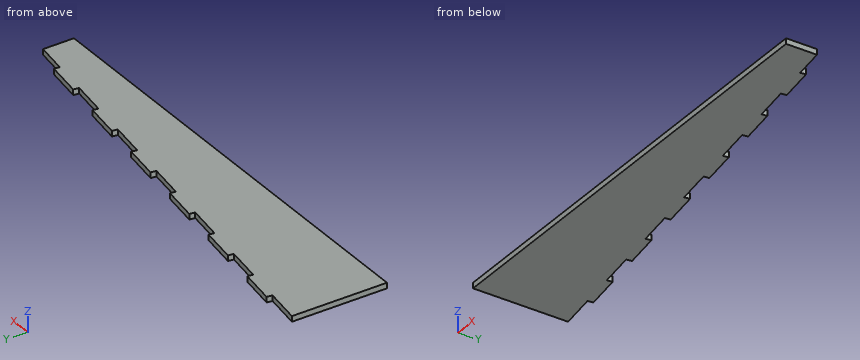
```python
from build123d import *

# Parameters (mm, degrees)
BOSS_EXTRU_1_DEPTH      = 3
ENL_V_MAT_EXTRU_1_DEPTH = 4


with BuildPart() as part:
    # Esquisse1 → Boss.-Extru.1 (new body)
    with BuildSketch(Plane.XY):
        Polygon((0, 0), (-255, 0), (-255, 55), (0, 19.9375), align=None)
    extrude(amount=BOSS_EXTRU_1_DEPTH)

    # Esquisse2 → Enlèv. mat.-Extru.1 (cut, through all)
    with BuildSketch(Plane.XY.offset(3)):
        Polygon((-235.186423203, 49.247406605), (-234.777768182, 52.219443125), (-255, 55), (-255, 51.971773415), align=None)
        Polygon((-195.150614588, 46.770709506), (-214.964191385, 49.495076315), (-215.372846406, 46.523039796), (-195.559269609, 43.798672986), align=None)
        Polygon((-155.523460994, 41.321975887), (-175.337037791, 44.046342696), (-175.745692812, 41.074306177), (-155.932116015, 38.349939367), align=None)
        Polygon((-115.8963074, 35.873242268), (-135.709884197, 38.597609077), (-136.118539219, 35.625572558), (-116.304962422, 32.901205748), align=None)
        Polygon((-76.269153806, 30.424508648), (-96.082730603, 33.148875458), (-96.491385625, 30.176838938), (-76.677808828, 27.452472129), align=None)
        Polygon((-36.642000213, 24.975775029), (-56.45557701, 27.700141839), (-56.864232031, 24.728105319), (-37.050655234, 22.00373851), align=None)
        Polygon((0, 19.9375), (-16.828423416, 22.25140822), (-17.237078437, 19.2793717), (0, 16.909273415), align=None)
    extrude(amount=-ENL_V_MAT_EXTRU_1_DEPTH, mode=Mode.SUBTRACT)


solid = part.part
```
Work out the finished part from the listing and answer in its coordinate system (mm). Coordinates: 2 decimals unless noted, no trailing zeros. Loops run counter-clockwise (first coordinate to the right, second up) from the corner with the lowest first, then second, coordinate; pieces in that order, holes last. Notation, with made-up numbers: M 84,47 L 104,47 A11 ccw 104,63 Z; hole C 54.5,40 d8. An arc over 180 degrees is marked long. Use CSV: the item, a comma, the result in double quotes. Start each with the question number.
(1) Find section A-A, the plane z = 1.6. Give the vertices of the cut face in (x, y), then the cut area to 3 significant figures.
(2) Find section C-C, the plane x = -238. Give the vertices of the cut face in (y, z).
(3) Consider line 1 (Y direction, x = -130, z = 2.35); line 2 (Y direction, x = -139, z = 0.5); line 3 (X direction, y = 21.5, z = 1.95). Determine where each line is inside the solid, lowest interval first.
(4) Given pin 1 Ø1 at (y, z) = (10, 1.5) entering from +X, flat-ended and moving along its own axis, determine where the tip first touches the part or whether it passes through.
(5) Find section B-B, the plane x = -204. Give the vertices of the cut face in (y, z), then the cut area to 3 significant figures.
Recorded:
1,outline,"M -255,0 L 0,0 L 0,16.91 L -17.24,19.28 L -16.83,22.25 L -36.64,24.98 L -37.05,22 L -56.86,24.73 L -56.46,27.7 L -76.27,30.42 L -76.68,27.45 L -96.49,30.18 L -96.08,33.15 L -115.9,35.87 L -116.3,32.9 L -136.12,35.63 L -135.71,38.6 L -155.52,41.32 L -155.93,38.35 L -175.75,41.07 L -175.34,44.05 L -195.15,46.77 L -195.56,43.8 L -215.37,46.52 L -214.96,49.5 L -234.78,52.22 L -235.19,49.25 L -255,51.97 Z"
1,area,"9,140 mm^2"
2,outline,"M 0,0 L 49.63,0 L 49.63,3 L 0,3 Z"
3,line 1,"y = 0 to 34.78"
3,line 2,"y = 0 to 39.05"
3,line 3,"x = -255 to -16.93"
4,pin 1,"stops at x = 0"
5,outline,"M 0,0 L 44.96,0 L 44.96,3 L 0,3 Z"
5,area,"135 mm^2"
